from build123d import *

# Parameters (mm, degrees)
BOSS_EXTRUDE1_DEPTH = 64
SKETCH2_R           = 8
CUT_EXTRUDE1_DEPTH  = 64
CUT_EXTRUDE2_REACH  = 146
SKETCH4_R           = 3
CUT_EXTRUDE3_DEPTH  = 10


with BuildPart() as part:
    # Sketch1 → Boss-Extrude1 (new body)
    with BuildSketch(Plane.XY):
        Polygon((0, 0), (144, 0), (144, 52), (122, 52), (122, 16), (26, 16), (26, 52), (16, 52), (0, 36), align=None)
    extrude(amount=BOSS_EXTRUDE1_DEPTH)

    # Sketch2 → Cut-Extrude1 (cut)
    with BuildSketch(Plane(origin=(144, 0, 0), x_dir=(0, 0, -1), z_dir=(1, 0, 0))):
        with BuildLine():
            Line((-64, 52), (-64, 16))
            Line((-64, 16), (-60.891410649, 16))
            ThreePointArc((-60.891410649, 16), (-59.279511824, 16.469825663), (-58.172487288, 17.732145215))
            Line((-58.172487288, 17.732145215), (-46.500924593, 42.761892188))
            ThreePointArc((-46.500924593, 42.761892188), (-40.596793734, 49.494263133), (-32, 52))
            Line((-32, 52), (-64, 52))
        make_face()
        with BuildLine():
            Line((0, 52), (-32, 52))
            ThreePointArc((-32, 52), (-23.403206266, 49.494263133), (-17.499075407, 42.761892188))
            Line((-17.499075407, 42.761892188), (-5.827512712, 17.732145215))
            ThreePointArc((-5.827512712, 17.732145215), (-4.720488176, 16.469825663), (-3.108589351, 16))
            Line((-3.108589351, 16), (0, 16))
            Line((0, 16), (0, 52))
        make_face()
        with Locations((-32, 36)):
            Circle(SKETCH2_R)
    extrude(amount=-CUT_EXTRUDE1_DEPTH, mode=Mode.SUBTRACT)

    # Sketch3 → Cut-Extrude2 (cut, up to next)
    with BuildSketch(Plane(origin=(144, 0, 0), x_dir=(0, 0, -1), z_dir=(1, 0, 0)), mode=Mode.PRIVATE) as cut_extrude2_sk1:
        Polygon((-48, 0), (-16, 0), (-16, 7), (-24, 7), (-24, 16), (-40, 16), (-40, 7), (-48, 7), align=None)
    cut_extrude2_tool1 = extrude(cut_extrude2_sk1.sketch, amount=-CUT_EXTRUDE2_REACH, mode=Mode.PRIVATE) & part.part
    add(cut_extrude2_tool1.solids().sort_by_distance((144, 6.630435, 32))[0], mode=Mode.SUBTRACT)

    # Sketch4 → Cut-Extrude3 (cut)
    with BuildSketch(Plane.XZ):
        with Locations((36, 54)):
            Circle(SKETCH4_R)
        with Locations((106, 54)):
            Circle(SKETCH4_R)
        with Locations((36, 10)):
            Circle(SKETCH4_R)
        with Locations((106, 10)):
            Circle(SKETCH4_R)
    extrude(amount=-CUT_EXTRUDE3_DEPTH, mode=Mode.SUBTRACT)


solid = part.part
Could you check a few things on this model? Use its own coordinates, in mm. A direction names the side the tool comes from. Coordinates: 2 decimals unless noted, no trailing zeros. Order: outer loops, then holes, each group sorted by start corner. A loop starts at its lowest first (then second) coordinate and runs counter-clockwise, first axis right, second up. Notation, with made-up numbers: (11, 32) -> (63, 32) arc R10 cw to (63, 51) -> close; hole circle Ø9 at (82.25, -26). An arc over 180 degrees is marked (long way). One line per item, written item: value. Start each with the question number.
1) Imagine slicing it at B-B on y = 49. List the corners of the cut face in (x, z) for me.
2) Imagine slicing it at D-D on z = 36. List the corners of the cut face in (x, y) for me.
3) If I drill on L1, parallel to Z at x = 106, y = 5.75; L2, parallel to X at y = 17.5, z = 23; L3, parallel to Z at x = 65.5, y = 6, over which ranges is the centre line in solid material (lowest first)? Write a range as [from, to].
4) I'm going to push flat-ended pins straight in: pin 1 (17.5 mm diameter, centred on x = 16.5, z = 29, fed in from -Y); pin 2 (6 mm diameter, centred on y = 6, z = 21, fed in from -X); pin 3 (5 mm diameter, centred on x = 36, z = 54, fed in from +Y); pin 4 (3 mm diameter, centred on x = 128, z = 15.5, fed in from +Y). Where does each tip first touch, or does it pass through?
5) We'd pull the mould along X, two halves only. Please class faces 1 (the flat face through (26, 34, 32)), 2 (the flat face through (55, 15, 0)), 3 (the flat face through (36, 10, 54)): +X half, -X half, draft (parallel to the pull), parting line (faces both ways), or undercut.
6) Imagine slicing it at C-C on y = 38.5. List the corners of the cut face in (x, z) for me.
7) Which directions (+Z, -Z, +X, -X, +Y, -Y) give clear straight access to the entire face, cutting with the end or side of a thin tool? Please do faces 4 (the cylindrical face through (133.2, 41.4, 37.9)), 5 (the flat face through (71, 0, 8)), 6 (the cylindrical face through (133.15, 16.48, 4.74)), 7 (the flat face through (73, 7, 20)), 8 (the cylindrical face through (33, 5, 10)).
8) Imagine slicing it at A-A on x = 106. List the corners of the cut face in (y, z) for me.
Answer list:
1. outline: (13, 0) -> (26, 0) -> (26, 64) -> (13, 64) -> close; (122, 22.67) -> (144, 22.67) -> (144, 41.33) -> (122, 41.33) -> close
2. outline: (0, 16) -> (26, 16) -> (26, 52) -> (16, 52) -> (0, 36) -> close; (122, 16) -> (144, 16) -> (144, 29.07) -> (122, 29.07) -> close; (122, 42.93) -> (144, 42.93) -> (144, 51.49) -> (122, 51.49) -> close
3. L1: z = [0, 7], [13, 16], [48, 51], [57, 64]
3. L2: x = [0, 26], [122, 144]
3. L3: z = [0, 16], [48, 64]
4. pin 1: stops at y = 7
4. pin 2: stops at x = 0
4. pin 3: stops at y = 16
4. pin 4: stops at y = 41.69
5. face 1: undercut
5. face 2: draft
5. face 3: undercut
6. outline: (2.5, 0) -> (26, 0) -> (26, 64) -> (2.5, 64) -> close; (122, 15.51) -> (144, 15.51) -> (144, 24.4) -> (122, 24.4) -> close; (122, 39.6) -> (144, 39.6) -> (144, 48.49) -> (122, 48.49) -> close
7. face 4: +X
7. face 5: +Z, -Z, +X, -X, -Y
7. face 6: -Z, +X, +Y
7. face 7: +X, -X, -Y
7. face 8: -Y
8. outline: (0, 0) -> (16, 0) -> (16, 24) -> (7, 24) -> (7, 16) -> (0, 16) -> (0, 13) -> (10, 13) -> (10, 7) -> (0, 7) -> close; (0, 48) -> (7, 48) -> (7, 40) -> (16, 40) -> (16, 64) -> (0, 64) -> (0, 57) -> (10, 57) -> (10, 51) -> (0, 51) -> close
